Read the model definition and answer for the solid it produces. Units are mm, in the model's axes. A direction names the side the tool comes from. Give positions to 0.01 mm unless a question says otherwise; leave off trailing zeros. Order: outer loops, then holes, each group sorted by start corner. A loop starts at its lowest first (then second) coordinate and runs counter-clockwise, first axis right, second up. Notation, with made-up numbers: (61, 27.25) - (76, 27.25) arc R32 ccw to (76, 66.25) - close; hole circle Ø2 at (1.25, 20). An arc over 180 degrees is marked (long way). Return JSON: item names as keys, results as strings.
```python
from build123d import *

# Parameters (mm, degrees)
SKETCH1_W           = 40
SKETCH1_H           = 300
BOSS_EXTRUDE1_DEPTH = 5
SKETCH2_W           = 30
SKETCH2_H           = 30
BOSS_EXTRUDE2_DEPTH = 150
SKETCH3_R           = 5
CUT_EXTRUDE2_DEPTH  = 5
SKETCH6_R           = 5
CUT_EXTRUDE3_DEPTH  = 5


with BuildPart() as part:
    # Sketch1 → Boss-Extrude1 (new body)
    with BuildSketch(Plane(origin=(0, 0, 0), x_dir=(1, 0, 0), z_dir=(0, 1, 0))):
        Rectangle(SKETCH1_W, SKETCH1_H)
    extrude(amount=BOSS_EXTRUDE1_DEPTH)

    # Sketch2 → Boss-Extrude2 (add)
    with BuildSketch(Plane(origin=(0, 5, 0), x_dir=(1, 0, 0), z_dir=(0, 1, 0))):
        with Locations((0, 65)):
            Rectangle(SKETCH2_W, SKETCH2_H)
        with Locations((0, -65)):
            Rectangle(SKETCH2_W, SKETCH2_H)
    extrude(amount=BOSS_EXTRUDE2_DEPTH)

    # Sketch3 → Cut-Extrude2 (cut)
    with BuildSketch(Plane(origin=(0, 5, 0), x_dir=(1, 0, 0), z_dir=(0, 1, 0))):
        with Locations(Location((-0.022747462, 135, 0), (0, 0, 270))):
            Circle(SKETCH3_R)
    extrude(amount=-CUT_EXTRUDE2_DEPTH, mode=Mode.SUBTRACT)

    # Sketch6 → Cut-Extrude3 (cut)
    with BuildSketch(Plane(origin=(0, 5, 0), x_dir=(1, 0, 0), z_dir=(0, 1, 0))):
        with Locations(Location((0.036186428, -135, 0), (0, 0, 270))):
            Circle(SKETCH6_R)
    extrude(amount=-CUT_EXTRUDE3_DEPTH, mode=Mode.SUBTRACT)


solid = part.part
```
Q1. For faces 1 (the flat face through (15, 79, 65)), 2 (the flat face through (0, 79, -80)), 3 (the flat face through (-15, 79, -65)), determine the directions among +Z, -Z, +X, -X, +Y, -Y from which every point of the face is accessible in a straight line to the end or side of a thin tool.
Values:
{"face 1": "+Z, -Z, +X, +Y", "face 2": "-Z, +X, -X, +Y", "face 3": "+Z, -Z, -X, +Y"}
Q2. A cutting plane is placed at C-C (x = -9.5). Write down the section's boundary in (y, z), and give its area (3 significant figures).
Values:
{"outline": "(0, -150) - (5, -150) - (5, -80) - (155, -80) - (155, -50) - (5, -50) - (5, 50) - (155, 50) - (155, 80) - (5, 80) - (5, 150) - (0, 150) - close", "area": "10,500 mm²"}
Q3. A cutting plane is placed at B-B (y = 83). Write down the section's boundary in (x, z), and give its area (3 significant figures).
Values:
{"outline": "(-15, -80) - (15, -80) - (15, -50) - (-15, -50) - close; (-15, 50) - (15, 50) - (15, 80) - (-15, 80) - close", "area": "1,800 mm²"}
Q4. A cutting plane is placed at D-D (z = -61). Write down the section's boundary in (x, y), and give its area (3 significant figures).
Values:
{"outline": "(-20, 0) - (20, 0) - (20, 5) - (15, 5) - (15, 155) - (-15, 155) - (-15, 5) - (-20, 5) - close", "area": "4,700 mm²"}
Q5. Determine the mould class of faces 4 (the flat face through (0, 79, 80)), 5 (the flat face through (0, 79, 50)), 6 (the flat face through (15, 79, -65)), 7 (the cylindrical face through (1.48, 2.54, -130.23)) for opening direction Z: released by +Z, released by -Z, zero draft, split by the parting line, or undercut.
Values:
{"face 4": "released by +Z", "face 5": "undercut", "face 6": "zero draft", "face 7": "undercut"}
Q6. Given pin 1 (24 mm diameter, centred on y = 60, z = 70, fed in from +X); pin 2 (1.5 mm diameter, centred on x = 13.5, y = 58.5, fed in from +Z); pin 3 (1 mm diameter, centred on x = 6.5, y = 127, fed in from -Z), each flat-ended and moving along its own axis, determine where each tip first touches the part or whether it passes through.
Values:
{"pin 1": "stops at x = 15", "pin 2": "stops at z = 80", "pin 3": "stops at z = -80"}
Q7. A cutting plane is placed at A-A (z = -135). Write down the section's boundary in (x, y), and give its area (3 significant figures).
Values:
{"outline": "(-20, 0) - (-5.02, 0) - (-5.02, 5) - (-20, 5) - close; (4.98, 0) - (20, 0) - (20, 5) - (4.98, 5) - close", "area": "150 mm²"}
Q8. Consider L1, parallel to Z at x = -7, y = 111.5; L2, parallel to X at y = 3, z = 135; L3, parallel to Y at x = -7, z = 42. Determine where each line is inside the solid, lowest interval first.
Values:
{"L1": "z = -80 to -50, 50 to 80", "L2": "x = -20 to -4.96, 5.04 to 20", "L3": "y = 0 to 5"}
